Design review of the part built by this model. Coordinates are the model's own, in mm. Give positions to 0.01 mm unless a question says otherwise; leave off trailing zeros. Loops run counter-clockwise (first coordinate to the right, second up) from the corner with the lowest first, then second, coordinate; pieces in that order, holes last.
from build123d import *

# Parameters (mm, degrees)
SKETCH2_W           = 105
SKETCH2_H           = 60
BOSS_EXTRUDE1_DEPTH = 3
SKETCH3_R           = 1.5
SKETCH3_R_2         = 2
CUT_EXTRUDE1_DEPTH  = 4
CUT_EXTRUDE2_DEPTH  = 4


with BuildPart() as part:
    # Sketch2 → Boss-Extrude1 (new body)
    with BuildSketch(Plane.XY):
        Rectangle(SKETCH2_W, SKETCH2_H)
    extrude(amount=BOSS_EXTRUDE1_DEPTH)

    # Sketch3 → Cut-Extrude1 (cut, through all)
    with BuildSketch(Plane.XY.offset(3)):
        with Locations((-47.5, 25)):
            Circle(SKETCH3_R)
        with Locations((47.5, 25)):
            Circle(SKETCH3_R)
        with Locations((47.5, -25)):
            Circle(SKETCH3_R)
        with Locations((-47.5, -25)):
            Circle(SKETCH3_R)
        with Locations((-42.5, 0)):
            Circle(SKETCH3_R_2)
        with Locations((-22.5, 0)):
            Circle(SKETCH3_R_2)
        with Locations((7.5, 0)):
            Circle(SKETCH3_R_2)
    extrude(amount=-CUT_EXTRUDE1_DEPTH, mode=Mode.SUBTRACT)

    # Sketch4 → Cut-Extrude2 (cut, through all)
    with BuildSketch(Plane.XY.offset(3)):
        with BuildLine():
            Line((-41, 25), (-25.75, 25))
            Line((-25.75, 25), (-25.75, 5.629165125))
            ThreePointArc((-25.75, 5.629165125), (-27.096194078, 4.596194078), (-28.129165125, 3.25))
            Line((-28.129165125, 3.25), (-36.870834875, 3.25))
            ThreePointArc((-36.870834875, 3.25), (-40.959393148, 6.314786657), (-46, 5.477225575))
            Line((-46, 5.477225575), (-46, 18.67544468))
            ThreePointArc((-46, 18.67544468), (-42.400980486, 20.968871126), (-41, 25))
        make_face()
        with BuildLine():
            Line((-19.25, 25), (4.25, 25))
            Line((4.25, 25), (4.25, 5.629165125))
            ThreePointArc((4.25, 5.629165125), (2.903805922, 4.596194078), (1.870834875, 3.25))
            Line((1.870834875, 3.25), (-16.870834875, 3.25))
            ThreePointArc((-16.870834875, 3.25), (-17.903805922, 4.596194078), (-19.25, 5.629165125))
            Line((-19.25, 5.629165125), (-19.25, 25))
        make_face()
        with BuildLine():
            Line((46, 18.67544468), (46, 3.25))
            Line((46, 3.25), (13.129165125, 3.25))
            ThreePointArc((13.129165125, 3.25), (12.096194078, 4.596194078), (10.75, 5.629165125))
            Line((10.75, 5.629165125), (10.75, 25))
            Line((10.75, 25), (41, 25))
            ThreePointArc((41, 25), (42.400980486, 20.968871126), (46, 18.67544468))
        make_face()
        with BuildLine():
            Line((46, -3.25), (13.129165125, -3.25))
            ThreePointArc((13.129165125, -3.25), (12.096194078, -4.596194078), (10.75, -5.629165125))
            Line((10.75, -5.629165125), (10.75, -25))
            Line((10.75, -25), (41, -25))
            ThreePointArc((41, -25), (42.400980486, -20.968871126), (46, -18.67544468))
            Line((46, -18.67544468), (46, -3.25))
        make_face()
        with BuildLine():
            Line((-16.870834875, -3.25), (1.870834875, -3.25))
            ThreePointArc((1.870834875, -3.25), (2.903805922, -4.596194078), (4.25, -5.629165125))
            Line((4.25, -5.629165125), (4.25, -25))
            Line((4.25, -25), (-19.25, -25))
            Line((-19.25, -25), (-19.25, -5.629165125))
            ThreePointArc((-19.25, -5.629165125), (-17.903805922, -4.596194078), (-16.870834875, -3.25))
        make_face()
        with BuildLine():
            Line((-46, -18.67544468), (-46, -5.477225575))
            ThreePointArc((-46, -5.477225575), (-40.959393148, -6.314786657), (-36.870834875, -3.25))
            Line((-36.870834875, -3.25), (-28.129165125, -3.25))
            ThreePointArc((-28.129165125, -3.25), (-27.096194078, -4.596194078), (-25.75, -5.629165125))
            Line((-25.75, -5.629165125), (-25.75, -25))
            Line((-25.75, -25), (-41, -25))
            ThreePointArc((-41, -25), (-42.400980486, -20.968871126), (-46, -18.67544468))
        make_face()
    extrude(amount=-CUT_EXTRUDE2_DEPTH, mode=Mode.SUBTRACT)


solid = part.part
Q1. Take a section at C-C (x = -22.5). Give the boundary of the cut face in (y, z), plus the area to 3 significant figures.
Results:
outline: (-30, 0) - (-2, 0) - (-2, 3) - (-30, 3) - close; (2, 0) - (30, 0) - (30, 3) - (2, 3) - close
area: 168 mm2
Q2. Take a section at B-B (x = 14.5). Give the boundary of the cut face in (y, z).
Results:
outline: (-30, 0) - (-25, 0) - (-25, 3) - (-30, 3) - close; (-3.25, 0) - (3.25, 0) - (3.25, 3) - (-3.25, 3) - close; (25, 0) - (30, 0) - (30, 3) - (25, 3) - close
Q3. Take a section at D-D (z = 2.1). Give the number of separate pieces and of enclosed holes in the cut face, plus the area to 3 significant figures.
Results:
separate pieces: 1
enclosed holes: 13
area: 2,960 mm2
Q4. Insertion check: pin 1 (2.5 mm diameter, centred on x = 47.5, y = -25, fed in from +Z). The pin has a flat end and moves straight along its axis. Give the tip position at first contact, or say it passes through.
Results:
pin 1: passes through
Q5. Draft analysis for pull direction Y (two halves, no side actions). For faces 1 (the face through (10.75, 15, 2)), 2 (the face through (-12, 0, 3)), state which applies: pulls with the +Y half, pulls with the -Y half, needs draft (parallel to the pull), parting line crosses it, or undercut.
Results:
face 1: undercut
face 2: needs draft
Q6. Wall thickness on line 1 (X direction, y = 8, z = 1); line 2 (Y direction, x = 38, z = 0.3); line 3 (Y direction, x = 47.5, z = 0.85): over which ranges is each line inside the solid? List them lowest first.
Results:
line 1: x = -52.5 to -46, -25.75 to -19.25, 4.25 to 10.75, 46 to 52.5
line 2: y = -30 to -25, -3.25 to 3.25, 25 to 30
line 3: y = -30 to -26.5, -23.5 to 23.5, 26.5 to 30
Q7. Take a section at A-A (y = 0). Give the boundary of the cut face in (x, z).
Results:
outline: (-52.5, 0) - (-44.5, 0) - (-44.5, 3) - (-52.5, 3) - close; (-40.5, 0) - (-24.5, 0) - (-24.5, 3) - (-40.5, 3) - close; (-20.5, 0) - (5.5, 0) - (5.5, 3) - (-20.5, 3) - close; (9.5, 0) - (52.5, 0) - (52.5, 3) - (9.5, 3) - close
